Check sheet for the drawn part. Datum: minimum x, y, z corner. Units: mm. A direction names the side the tool comes from. Give positions to 0.01 mm unless a question says otherwise; leave off trailing zeros. Order: outer loops, then holes, each group sorted by start corner. A loop starts at its lowest first (then second) coordinate and runs counter-clockwise, first axis right, second up. Notation, with made-up numbers: (-3.75, 50.5) -> (26.25, 50.5) arc R14 ccw to (26.25, 67.5) -> close; hole circle Ø2 at (60, -23.5). An arc over 180 degrees is marked (long way). Answer in a Markdown table with one row per item. Add a question column.
(1) Cross-section at C-C (z = 20). Record the cut outline in (x, y) (3 decimals).
(2) Go/stop test with flat-tipped pins: pin 1 (1 mm diameter, centred on x = 7, y = 0.5, fed in from -Z); pin 2 (0.8 mm diameter, centred on y = 1.5, z = 13.5, fed in from +X); pin 3 (1.5 mm diameter, centred on x = 6, y = 5.5, fed in from -Z). Record where each tip stops, or that it passes through.
(3) Thickness scan on L1, parallel to X at y = 2.5, z = 15.5; L2, parallel to X at y = 1.25, z = 22. Record the ranges inside material, lowest first. Write a range as [from, to].
(4) Set-up check for the marked faces 1, 2 and 3: record each of +Z, -Z, +X, -X, +Y, -Y from which the full face is reachable in a straight line by a thin tool's end or side.
(5) Cross-section at D-D (y = 5.75). Record the cut outline in (x, z), then the cut area to 3 significant figures.
(6) Cross-section at B-B (z = 16). Record the cut outline in (x, y) (3 decimals).
(7) Cross-section at A-A (x = 20). Record the cut outline in (y, z) (3 decimals).
(8) Release check for a two-part mould opening along X. For the marked faces 4, 5 and 6 record: released by +X, released by -X, zero draft, split by the parting line, or undercut.
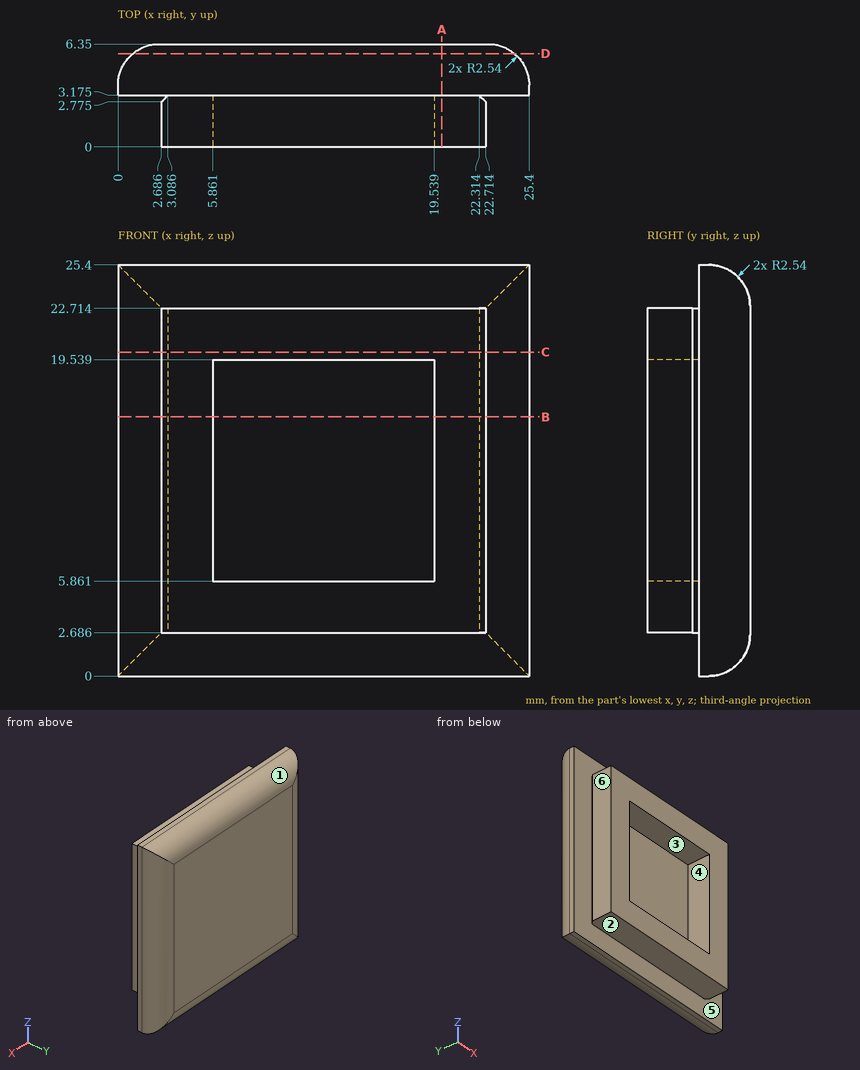
Answer below:
| question | item | result |
|---|---|---|
| 1 | outline | (0, 3.175) -> (3.086, 3.175) -> (2.686, 2.775) -> (2.686, 0) -> (22.714, 0) -> (22.714, 2.775) -> (22.314, 3.175) -> (25.4, 3.175) -> (25.4, 3.81) arc R2.54 ccw to (22.86, 6.35) -> (2.54, 6.35) arc R2.54 ccw to (0, 3.81) -> close |
| 2 | pin 1 | stops at z = 2.69 |
| 2 | pin 2 | stops at x = 22.71 |
| 2 | pin 3 | stops at z = 0.18 |
| 3 | L1 | x = [2.69, 5.86], [19.54, 22.71] |
| 3 | L2 | x = [2.69, 22.71] |
| 4 | face 1 | +Z, +X, -X, +Y |
| 4 | face 2 | -Z, +X, -X, -Y |
| 4 | face 3 | -Y |
| 5 | outline | (0.9, 0.9) -> (24.5, 0.9) -> (24.5, 24.5) -> (0.9, 24.5) -> close |
| 5 | area | 557 mm² |
| 6 | outline | (0, 3.175) -> (3.086, 3.175) -> (2.686, 2.775) -> (2.686, 0) -> (5.861, 0) -> (5.861, 3.175) -> (19.539, 3.175) -> (19.539, 0) -> (22.714, 0) -> (22.714, 2.775) -> (22.314, 3.175) -> (25.4, 3.175) -> (25.4, 3.81) arc R2.54 ccw to (22.86, 6.35) -> (2.54, 6.35) arc R2.54 ccw to (0, 3.81) -> close |
| 7 | outline | (0, 2.686) -> (3.175, 2.686) -> (3.175, 0) -> (3.81, 0) arc R2.54 ccw to (6.35, 2.54) -> (6.35, 22.86) arc R2.54 ccw to (3.81, 25.4) -> (3.175, 25.4) -> (3.175, 22.714) -> (0, 22.714) -> close |
| 8 | face 4 | undercut |
| 8 | face 5 | zero draft |
| 8 | face 6 | released by -X |
